Design review of the part built by this model. Coordinates are the model's own, in mm. A direction names the side the tool comes from. Coordinates: 2 decimals unless noted, no trailing zeros. Loops run counter-clockwise (first coordinate to the right, second up) from the corner with the lowest first, then second, coordinate; pieces in that order, holes last. Notation, with made-up numbers: (-8, -13.75) -> (43, -13.75) arc R23 cw to (43, 2.25) -> close; hole circle Ø11 at (11, 63). An arc over 180 degrees is marked (long way). Use CSV: the item, a comma, the result in double quotes.
```python
from build123d import *

# Parameters (mm, degrees)
BOSS_EXTRUDE1_DEPTH = 6
FILLET1_R           = 0.975
FILLET2_R           = 0.4


with BuildPart() as part:
    # Sketch1 → Boss-Extrude1 (new body)
    with BuildSketch(Plane.XY):
        with BuildLine():
            Line((-4, -4.95), (-4, 4.05))
            Line((-4, 4.05), (-2.05, 4.05))
            Line((-2.05, 4.05), (-2.05, 20.05))
            Line((-2.05, 20.05), (2.05, 20.05))
            Line((2.05, 20.05), (2.05, 4.05))
            Line((2.05, 4.05), (4, 4.05))
            Line((4, 4.05), (4, -4.95))
            Line((4, -4.95), (2.05, -4.95))
            Line((2.05, -4.95), (2.05, 0))
            ThreePointArc((2.05, 0), (0, 2.05), (-2.05, 0))
            Line((-2.05, 0), (-2.05, -4.95))
            Line((-2.05, -4.95), (-4, -4.95))
        make_face()
    extrude(amount=BOSS_EXTRUDE1_DEPTH)

    # Fillet1
    fillet1_edges = [part.edges().sort_by_distance(p)[0] for p in [
        (-4, -4.95, 3),
        (-4, 4.05, 3),
        (-2.05, 4.05, 3),
        (4, 4.05, 3),
        (4, -4.95, 3),
        (2.05, 4.05, 3),
        (-2.05, 20.05, 3),
        (2.05, 20.05, 3),
    ]]
    fillet(fillet1_edges, radius=FILLET1_R - 0.0001)  # a hair under: the kernel refuses the full size

    # Fillet2
    fillet2_edges = [part.edges().sort_by_distance(p)[0] for p in [
        (2.05, -4.95, 3),
        (-2.05, -4.95, 3),
    ]]
    fillet(fillet2_edges, radius=FILLET2_R)


solid = part.part
```
Item 1: To check wall thickness, follow line 1 along X through (y, z) = (-0.25, 4.35); line 2 along X through (y, z) = (18.5, 2.35); line 3 along Y through (x, z) = (0.5, 1.35). State the ranges of each line that lie inside material, in increasing order.
Checked values:
line 1,"-4 to -2.05, 2.05 to 4"
line 2,"-2.05 to 2.05"
line 3,"1.99 to 20.05"
Item 2: Add section C-C (x = 3.5). Give the boundary of the cut face in (y, z), then the cut area to 3 significant figures.
Checked values:
outline,"(-4.83, 0) -> (3.93, 0) -> (3.93, 6) -> (-4.83, 6) -> close"
area,"52.5 mm^2"
Item 3: Add section B-B (x = 0). Give the boundary of the cut face in (y, z).
Checked values:
outline,"(2.05, 0) -> (20.05, 0) -> (20.05, 6) -> (2.05, 6) -> close"
Item 4: Clearance check with a flat-ended pin moving along its axis: pin 1 (3 mm diameter, centred on y = 10, z = 3.5, fed in from -X). State where the tip first meets the part, or that it passes through.
Checked values:
pin 1,"x = -2.05"
Item 5: Draft analysis for pull direction X (two halves, no side actions). For faces 5 (the face through (-3.72, -4.66, 3.04)), 6 (the face through (1.76, 19.77, 3.04)), 7 (the face through (0.05, 2.05, 2.96)), state which applies: pulls with the +X half, pulls with the -X half, needs draft (parallel to the pull), parting line crosses it, or undercut.
Checked values:
face 5,"pulls with the -X half"
face 6,"pulls with the +X half"
face 7,"undercut"
Item 6: Machinability: for faces 1 (the face through (-2.05, -2, 3)), 2 (the face through (3.72, -4.66, 3.04)), 3 (the face through (-2.05, 12, 3)), 4 (the face through (2.05, 12, 3)), which of the approach directions +Z, -Z, +X, -X, +Y, -Y give a long, thin tool a straight path to every point of the face, cutting with its end or side? Answer none if there is none.
Checked values:
face 1,"+Z, -Z, -Y"
face 2,"+Z, -Z, +X, -Y"
face 3,"+Z, -Z, -X, +Y"
face 4,"+Z, -Z, +X, +Y"
